The figure shows three views and two pictorial views of one solid part (mm, origin at its lowest corner). Answer the questions. Give positions to 0.01 mm unless a question says otherwise; leave off trailing zeros. Loops run counter-clockwise (first coordinate to the right, second up) from the corner with the lowest first, then second, coordinate; pieces in that order, holes last.
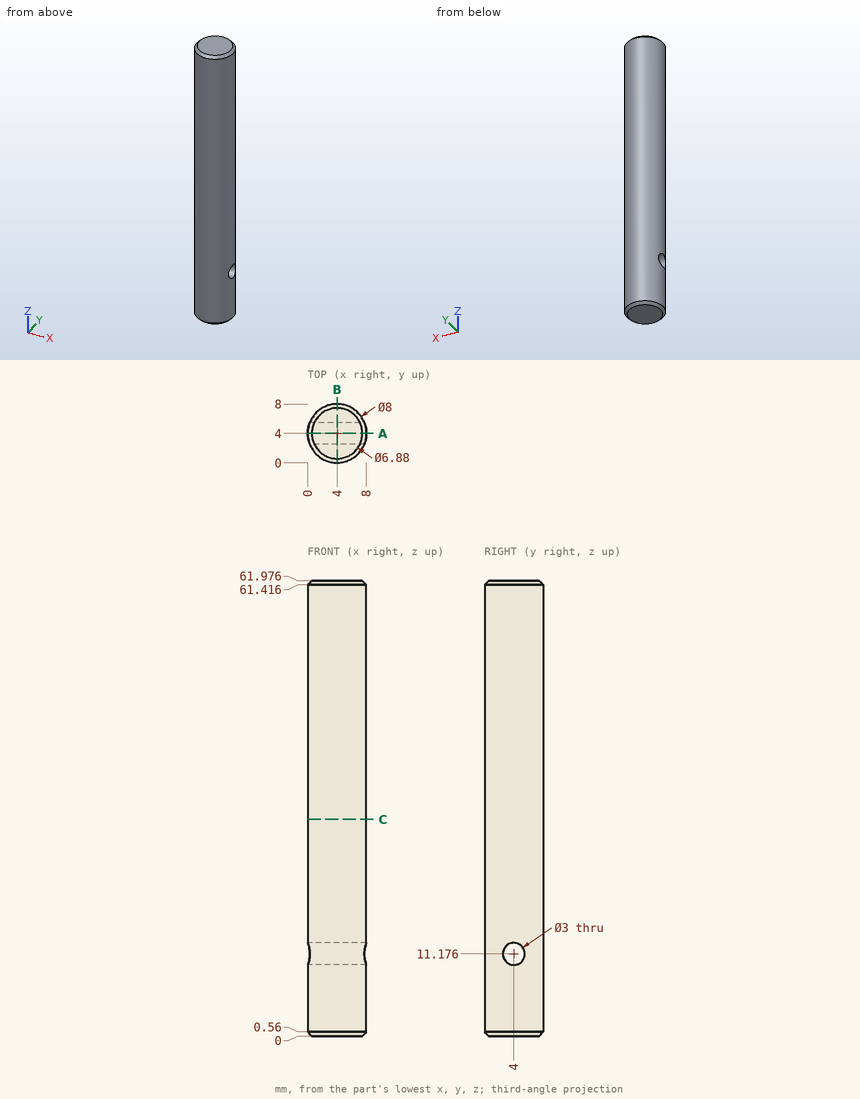
Q1. Consider line 1 along Z through (x, y) = (3.5, 4); line 2 along Z through (x, y) = (1, 2.75); line 3 along Y through (x, z) = (2.5, 11.5). Determine where each line is inside the solid, lowest interval first.
Q2. Section C-C on z = 29.5 is taken. Give the vertices of the cut face in (x, y).
Q3. Section B-B on x = 4 is taken. Give the vertices of the cut face in (y, z), plus the area to 3 significant figures.
Q4. Section A-A on y = 4 is taken. Give the vertices of the cut face in (x, z), plus the area to 3 significant figures.
Check result:
1. line 1: z = 0 to 9.68, 12.68 to 61.98
1. line 2: z = 0 to 10.35, 12.01 to 61.98
1. line 3: y = 0.29 to 2.54, 5.46 to 7.71
2. outline: circle Ø8 at (4, 4)
3. outline: (0, 0.56) - (0.56, 0) - (7.44, 0) - (8, 0.56) - (8, 61.42) - (7.44, 61.98) - (0.56, 61.98) - (0, 61.42) - close; hole circle Ø3 at (4, 11.18)
3. area: 488 mm2
4. outline: (0, 0.56) - (0.56, 0) - (7.44, 0) - (8, 0.56) - (8, 9.68) - (0, 9.68) - close; (0, 12.68) - (8, 12.68) - (8, 61.42) - (7.44, 61.98) - (0.56, 61.98) - (0, 61.42) - close
4. area: 471 mm2
